Geometry check sheet. Reference: the model listing, model coordinates, mm. Face numbers are marked on the shaded views. A direction names the side the tool comes from. Coordinates: 2 decimals unless noted, no trailing zeros. Loops run counter-clockwise (first coordinate to the right, second up) from the corner with the lowest first, then second, coordinate; pieces in that order, holes last.
Autodesk Inventor part; units mm, degrees
ref_plane "YZ Plane" through (0, 0, 0) normal (1, 0, 0) x (0, 1, 0)
ref_plane "XZ Plane" through (0, 0, 0) normal (0, 1, 0) x (-1, 0, 0)
ref_plane "XY Plane" through (0, 0, 0) normal (0, 0, 1) x (1, 0, 0)
sketch "Skizze1" plane through (0, 0, 0) normal (0, 0, 1) x (1, 0, 0)
  line L0 (30, -25) -> (-30, -25)
  line L1 (-30, -25) -> (-30, 25)
  line L2 (-30, 25) -> (30, 25)
  line L3 (30, 25) -> (30, -25)
  point P0 (0, 0)
  point P1 (-30, 0)
  point P2 (0, 25)
  dimension "d0" = 50
  dimension "d1" = 60
extrude "Extrusion1" add sketch "Skizze1" against normal blind 29.1
sketch "Skizze2" plane through (0, 0, 0) normal (0, 0, 1) x (1, 0, 0)
  line L0 (-30, -25) -> (30, -25)
  circle A0 centre (0, 6.981) radius 5
  point P0 (0, 0)
  dimension "d4" = 31.981
  dimension "d5" = 10
sketch "Skizze4" plane through (30, -25, 0) normal (1, 0, 0) x (0, 0, -1)
  line L0 (0, 0) -> (0, 50)
  line L1 (0, 0) -> (29.1, 0)
  line L2 (29.1, 0) -> (19.4, 0)
  line L3 (9.7, 0) -> (19.4, 0)
  line L4 (19.4, 0) -> (19.4, 1)
  line L5 (19.4, 1) -> (9.7, 1)
  line L6 (9.7, 1) -> (9.7, 0)
  point P0 (0, 25)
extrude "Extrusion3" add sketch "Skizze4" along normal blind 7
mirror "Spiegeln1" about plane through (0, 0, 0) normal (1, 0, 0) of "Extrusion3"
sketch "Skizze5" plane through (30, -24, -9.7) normal (0, 1, 0) x (1, 0, 0)
  line L0 (7, 0) -> (7, 9.7)
  line L1 (0, -9.7) -> (0, 19.4)
  line L2 (0, -9.7) -> (0, 0)
  line L3 (-60, 9.7) -> (-60, 0)
  line L4 (-60, 9.7) -> (-67, 9.7)
  line L5 (-67, 9.7) -> (-67, 0)
  point P0 (-30, -9.7)
  point P1 (3.5, 4.7412)
  point P2 (-63.5, 4.85)
sketch "Skizze6" plane through (-30, 25, 0) normal (0, 1, 0) x (1, 0, 0)
  line L0 (17.0015, 26.6738) -> (64.1972, 26.6738) construction
  line L1 (64.1972, 26.6738) -> (64.1972, 22.3208) construction
  line L2 (64.1972, 22.3208) -> (17.0015, 22.3208) construction
  line L3 (17.0015, 22.3208) -> (17.0015, 26.6738) construction
  point P0 (30, 0)
extrude "Extrusion4" add sketch "Skizze2" along normal blind 0.5
properties part number "Lenkmotor1" material "Gold"
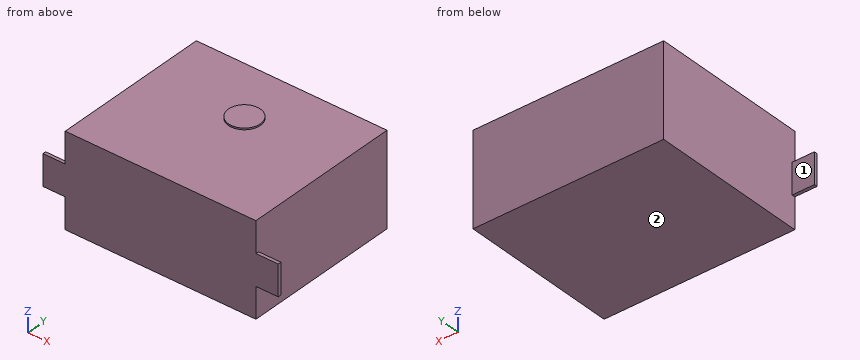
(1) Sectioned sample at C-C on y = 10. Record the cut outline in (x, z).
Findings:
outline: (-30, -29.1) - (30, -29.1) - (30, 0) - (3.99, 0) - (3.99, 0.5) - (-3.99, 0.5) - (-3.99, 0) - (-30, 0) - close
(2) Sectioned sample at B-B on x = -21.5. Record the cut outline in (y, z), and give its area (4 significant figures).
Findings:
outline: (-25, -29.1) - (25, -29.1) - (25, 0) - (-25, 0) - close
area: 1,455 mm2
(3) Sectioned sample at D-D on z = -2.75. Record the cut outline in (x, y), and give its area (3 significant figures).
Findings:
outline: (-30, -25) - (30, -25) - (30, 25) - (-30, 25) - close
area: 3,000 mm2
(4) Gauge pin test, flat ends, axial feed: pin 1 Ø1.1 at (x, y) = (35, -24.5) entering from -Z; pin 2 Ø2 at (y, z) = (-17, -5.5) entering from -X; pin 3 Ø1 at (y, z) = (-14, -11.5) entering from +X. Record the tip position at first contact, or that the pin passes through.
Findings:
pin 1: stops at z = -19.4
pin 2: stops at x = -30
pin 3: stops at x = 30
(5) Access from +Z, -Z, +X, -X, +Y, -Y to the whole of each face (thin tool, end or side, straight path). Record for the marked faces 1 and 2.
Findings:
face 1: +Z, -Z, -X, +Y
face 2: -Z, +X, -X, +Y, -Y
(6) Scan lines: L1, parallel to X at y = -6, z = -7.5; L2, parallel to Y at x = -33, z = -17.5; L3, parallel to Z at x = -13, y = 14. Record each from-to range of solid material in increasing order.
Findings:
L1: x = -30 to 30
L2: y = -25 to -24
L3: z = -29.1 to 0
(7) Sectioned sample at A-A on z = -13.5. Record the cut outline in (x, y), and give its area (3 significant figures).
Findings:
outline: (-37, -25) - (37, -25) - (37, -24) - (30, -24) - (30, 25) - (-30, 25) - (-30, -24) - (-37, -24) - close
area: 3,010 mm2
